Design review of the part shown in the three views and the two pictorial views. Dimensions are in mm from the part's minimum x, y and z. Give positions to 0.01 mm unless a question says otherwise; leave off trailing zeros. Order: outer loops, then holes, each group sorted by start corner. A loop starts at its lowest first (then second) coordinate and runs counter-clockwise, first axis right, second up. Notation, with made-up numbers: (66.25, 43) -> (105.25, 43) arc R18 ccw to (105.25, 55) -> close; hole circle Ø7 at (-17, -10.75). An arc over 180 degrees is marked (long way). Use one line per item in the form item = value.
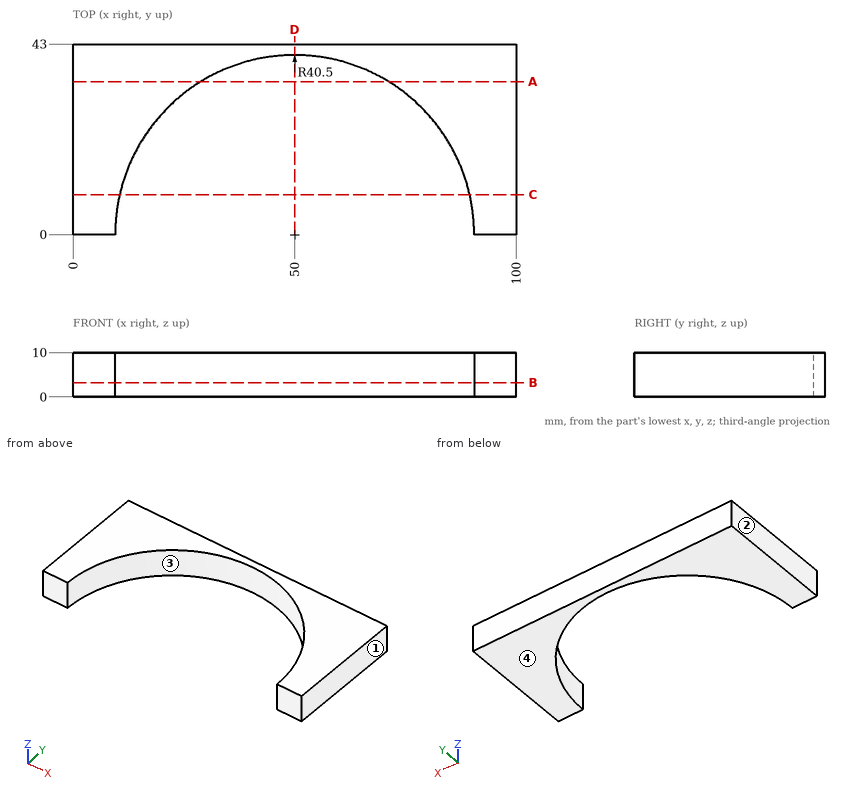
1. Add section B-B on z = 3.25. Give the boundary of the cut face in (x, y).
Values:
outline = (0, 0) -> (9.5, 0) arc R40.5 cw to (90.5, 0) -> (100, 0) -> (100, 43) -> (0, 43) -> close
2. Add section D-D on x = 50. Give the boundary of the cut face in (y, z).
Values:
outline = (40.5, 0) -> (43, 0) -> (43, 10) -> (40.5, 10) -> close
3. The part is to be moulded in two halves that separate along X. For the marked faces 1, 2, 3 and 4, say which applies: +X half, -X half, draft (parallel to the pull), parting line (faces both ways), or undercut.
Values:
face_1 = +X half
face_2 = -X half
face_3 = undercut
face_4 = draft
4. For L1, parallel to X at y = 9, z = 0.75; L2, parallel to X at y = 22.5, z = 1.75; L3, parallel to Y at x = 49, z = 8.5, list the stretches that pass through material, from the lowest coordinate up.
Values:
L1 = 0 to 10.51, 89.49 to 100
L2 = 0 to 16.33, 83.67 to 100
L3 = 40.49 to 43
5. Add section A-A on y = 34.5. Give the boundary of the cut face in (x, z), then the cut area to 3 significant figures.
Values:
outline = (0, 0) -> (28.79, 0) -> (28.79, 10) -> (0, 10) -> close; (71.21, 0) -> (100, 0) -> (100, 10) -> (71.21, 10) -> close
area = 576 mm^2
6. Add section C-C on y = 9. Give the boundary of the cut face in (x, z).
Values:
outline = (0, 0) -> (10.51, 0) -> (10.51, 10) -> (0, 10) -> close; (89.49, 0) -> (100, 0) -> (100, 10) -> (89.49, 10) -> close
7. For pin 1 Ø1.5 at (x, z) = (82.5, 6) entering from -Y, flat-tipped, find the tip position at first contact; note if it passes through.
Values:
pin_1 = 23.12
